Build history of the part. All positions in model axes, mm. Face numbers are marked on the shaded views. Give positions to 0.01 mm unless a question says otherwise; leave off trailing zeros. Order: outer loops, then holes, each group sorted by start corner. A loop starts at its lowest first (then second) coordinate and runs counter-clockwise, first axis right, second up. Notation, with made-up numbers: (15, 88.5) - (32, 88.5) arc R27 cw to (32, 125.5) - close; hole circle Ø6 at (77, 16). An arc over 180 degrees is marked (long way). Use a Markdown table: item, result. Add a question column.
(1) Slice it at B-B (x = 35). Write the cut outline in (y, z).
(2) Wall check: line 1 (X direction, y = 2, z = -5.75); line 2 (Y direction, x = 33, z = 0.25); line 3 (X direction, y = 1.5, z = -2.5). Give the ranges that are in metal, low to high.
(3) Mould opens along X. For the marked faces 1, 2 and 3 say: +X half, -X half, draft (parallel to the pull), parting line (faces both ways), or undercut.
(4) Slice it at D-D (z = -7.25). Write the cut outline in (x, y).
(5) Slice it at A-A (z = -4). Write the cut outline in (x, y).
(6) Slice it at C-C (y = -13). Write the cut outline in (x, z).
(7) Flat gauge pins, fed straight in: pin 1 (6 mm diameter, centred on x = -11.5, y = 8.5, fed in from -Z); pin 2 (5 mm diameter, centred on x = 13.5, z = -0.5, fed in from -Y); pin 3 (1.8 mm diameter, centred on y = -2, z = -3, fed in from +X); pin 4 (0.7 mm diameter, centred on x = -22, z = -3.5, fed in from -Y). Where does each tip first touch, or does it go through?
from build123d import *

# Parameters (mm, degrees)
SKETCH1_W           = 80
SKETCH1_H           = 40
BOSS_EXTRUDE1_DEPTH = 4
FILLET1_R           = 4
FILLET2_R           = 3
SKETCH2_W           = 74
SKETCH2_H           = 34
CUT_EXTRUDE1_DEPTH  = 1
BOSS_EXTRUDE2_DEPTH = 4
FILLET3_R           = 1
BOSS_EXTRUDE3_DEPTH = 9.5
LPATTERN1_COUNT     = 2
LPATTERN1_PITCH     = 40


with BuildPart() as part:
    # Sketch1 → Boss-Extrude1 (new body)
    with BuildSketch(Plane.XY):
        Rectangle(SKETCH1_W, SKETCH1_H)
    extrude(amount=BOSS_EXTRUDE1_DEPTH)

    # Fillet1
    fillet1_edges = [part.edges().sort_by_distance(p)[0] for p in [
        (-40, 20, 2),
        (40, 20, 2),
        (40, -20, 2),
        (-40, -20, 2),
    ]]
    fillet(fillet1_edges, radius=FILLET1_R)

    # Fillet2
    fillet2_edges = [part.edges().sort_by_distance(p)[0] for p in [
        (0, -20, 4),
        (-40, 0, 4),
        (40, 0, 4),
        (0, 20, 4),
        (-38.828427125, 18.828427125, 4),
        (38.828427125, 18.828427125, 4),
        (38.828427125, -18.828427125, 4),
        (-38.828427125, -18.828427125, 4),
    ]]
    fillet(fillet2_edges, radius=FILLET2_R)

    # Sketch2 → Cut-Extrude1 (cut)
    with BuildSketch(Plane(origin=(0, 0, 0), x_dir=(-1, 0, 0), z_dir=(0, 0, -1))):
        Rectangle(SKETCH2_W, SKETCH2_H)
    extrude(amount=-CUT_EXTRUDE1_DEPTH, mode=Mode.SUBTRACT)

    # Sketch3 → Boss-Extrude2 (add, symmetric)
    with BuildSketch(Plane(origin=(0, 0, 0), x_dir=(0, 0, -1), z_dir=(0, 1, 0))):
        Polygon((0, -37), (3, -38.091910703), (3, -39.7), (0, -39.7), align=None)
    extrude(amount=BOSS_EXTRUDE2_DEPTH, both=True)

    # Fillet3
    fillet3_edges = [part.edges().sort_by_distance(p)[0] for p in [
        (38.895955351, -4, -3),
        (38.895955351, 4, -3),
    ]]
    fillet(fillet3_edges, radius=FILLET3_R)

    # Sketch4 → Boss-Extrude3 (add)
    with BuildSketch(Plane(origin=(0, 0, 1), x_dir=(-1, 0, 0), z_dir=(0, 0, -1))):
        with BuildLine():
            Line((-23.301893396, -1), (-21, -1))
            Line((-21, -1), (-21, -3.301893396))
            ThreePointArc((-21, -3.301893396), (-20, -3.45), (-19, -3.301893396))
            Line((-19, -3.301893396), (-19, -1))
            Line((-19, -1), (-16.698106604, -1))
            ThreePointArc((-16.698106604, -1), (-16.55, 0), (-16.698106604, 1))
            Line((-16.698106604, 1), (-19, 1))
            Line((-19, 1), (-19, 3.301893396))
            ThreePointArc((-19, 3.301893396), (-20, 3.45), (-21, 3.301893396))
            Line((-21, 3.301893396), (-21, 1))
            Line((-21, 1), (-23.301893396, 1))
            ThreePointArc((-23.301893396, 1), (-23.45, 0), (-23.301893396, -1))
        make_face()
    boss_extrude3 = extrude(amount=BOSS_EXTRUDE3_DEPTH)

    # Sketch5 → Cut-Revolve1 (revolve, cut)
    with BuildSketch(Plane(origin=(0, 0, 0), x_dir=(0, 0, -1), z_dir=(0, 1, 0))):
        with BuildLine():
            Line((5.5, -16.55), (8.5, -16.55))
            Line((8.5, -16.55), (8.5, -17.498530758))
            ThreePointArc((8.5, -17.498530758), (8.383022222, -17.177136953), (8.086824089, -17.006126881))
            Line((8.086824089, -17.006126881), (5.5, -16.55))
        make_face()
    cut_revolve1 = revolve(axis=Axis((20, 0, 1), (0, 0, -1)), mode=Mode.SUBTRACT)

    # LPattern1: Boss-Extrude3, Cut-Revolve1 ×2
    with Locations(*[(-i * LPATTERN1_PITCH, 0, 0) for i in range(1, LPATTERN1_COUNT)]):
        add(boss_extrude3)
        add(cut_revolve1, mode=Mode.SUBTRACT)


solid = part.part
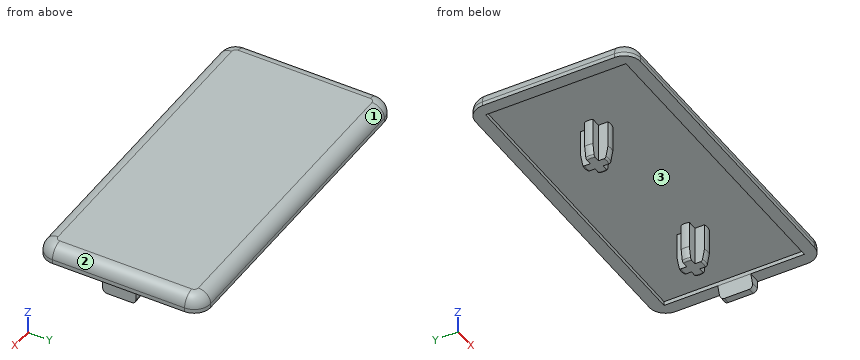
Solution:
| question | item | result |
|---|---|---|
| 1 | outline | (-20, 0) - (-17, 0) - (-17, 1) - (17, 1) - (17, 0) - (20, 0) - (20, 1) arc R3 ccw to (17, 4) - (-17, 4) arc R3 ccw to (-20, 1) - close |
| 2 | line 1 | -21 to -19, 19 to 21 |
| 2 | line 2 | -20 to -17, 17 to 20 |
| 2 | line 3 | -21 to -19, 19 to 21, 37.91 to 39.7 |
| 3 | face 1 | draft |
| 3 | face 2 | +X half |
| 3 | face 3 | undercut |
| 4 | outline | (-22.98, -1) - (-21, -1) - (-21, -2.98) arc R3.14 ccw to (-19, -2.98) - (-19, -1) - (-17.02, -1) arc R3.14 ccw to (-17.02, 1) - (-19, 1) - (-19, 2.98) arc R3.14 ccw to (-21, 2.98) - (-21, 1) - (-22.98, 1) arc R3.14 ccw to start; (17.02, -1) - (19, -1) - (19, -2.98) arc R3.14 ccw to (21, -2.98) - (21, -1) - (22.98, -1) arc R3.14 ccw to (22.98, 1) - (21, 1) - (21, 2.98) arc R3.14 ccw to (19, 2.98) - (19, 1) - (17.02, 1) arc R3.14 ccw to start |
| 5 | outline | (-23.3, -1) - (-21, -1) - (-21, -3.3) arc R3.45 ccw to (-19, -3.3) - (-19, -1) - (-16.7, -1) arc R3.45 ccw to (-16.7, 1) - (-19, 1) - (-19, 3.3) arc R3.45 ccw to (-21, 3.3) - (-21, 1) - (-23.3, 1) arc R3.45 ccw to start; (16.7, -1) - (19, -1) - (19, -3.3) arc R3.45 ccw to (21, -3.3) - (21, -1) - (23.3, -1) arc R3.45 ccw to (23.3, 1) - (21, 1) - (21, 3.3) arc R3.45 ccw to (19, 3.3) - (19, 1) - (16.7, 1) arc R3.45 ccw to start |
| 6 | outline | (-40, 0) - (-37, 0) - (-37, 1) - (37, 1) - (37, 0) - (40, 0) - (40, 1) arc R3 ccw to (37, 4) - (-37, 4) arc R3 ccw to (-40, 1) - close |
| 7 | pin 1 | z = 1 |
| 7 | pin 2 | y = -20 |
| 7 | pin 3 | x = 39.7 |
| 7 | pin 4 | y = -1 |
